```python
from build123d import *

# Parameters (mm, degrees)
BOSS_EXTRUDE1_DEPTH             = 5
F_3_0_3_DIAMETER_HOLE1_D        = 3
F_3_0_3_DIAMETER_HOLE1_DEPTH    = 6
F_3_0_3_DIAMETER_HOLE1_TIP      = 0.901290929
SKETCH6_W                       = 36
SKETCH6_H                       = 124
CUT_EXTRUDE1_DEPTH              = 3
SKETCH9_W                       = 20
SKETCH9_H                       = 45
CUT_EXTRUDE3_DEPTH              = 6
M3X0_5_TAPPED_HOLE1_D           = 2.5
M3X0_5_TAPPED_HOLE1_DEPTH       = 5
M3X0_5_TAPPED_HOLE1_CSINK_D     = 3.05
M3X0_5_TAPPED_HOLE1_CSINK_ANGLE = 90


with BuildPart() as part:
    # Sketch3 → Boss-Extrude1 (new body)
    with BuildSketch(Plane(origin=(0, -40, 0), x_dir=(-1, 0, 0), z_dir=(0, -1, 0))):
        Polygon((18.468579028, -110), (85.532661839, -110), (127, -68.532661839), (127, -18.529510204), (108.472719443, 10), (-4.471478576, 10), (-23, -18.531420972), (-23, -68.531420972), align=None)
    extrude(amount=BOSS_EXTRUDE1_DEPTH)

    # Ø3.0 (3) Diameter Hole1
    with Locations(Plane(origin=(0, -45, 0), x_dir=(-1, 0, 0), z_dir=(0, -1, 0))):
        with Locations((8.156954779, -77.608240604), (95.838195646, -77.608240604), (103.995150425, 0), (0, 0)):
            Hole(F_3_0_3_DIAMETER_HOLE1_D / 2, depth=F_3_0_3_DIAMETER_HOLE1_DEPTH)
            with Locations((0, 0, -(F_3_0_3_DIAMETER_HOLE1_DEPTH + F_3_0_3_DIAMETER_HOLE1_TIP / 2))):  # 118° drill point
                Cone(0, F_3_0_3_DIAMETER_HOLE1_D / 2, F_3_0_3_DIAMETER_HOLE1_TIP, mode=Mode.SUBTRACT)

    # Sketch6 → Cut-Extrude1 (cut)
    with BuildSketch(Plane(origin=(0, -45, 0), x_dir=(-1, 0, 0), z_dir=(0, -1, 0))):
        with Locations((52, -55)):
            Rectangle(SKETCH6_W, SKETCH6_H)
    extrude(amount=-CUT_EXTRUDE1_DEPTH, mode=Mode.SUBTRACT)

    # Sketch9 → Cut-Extrude3 (cut, through all)
    with BuildSketch(Plane(origin=(0, -45, 0), x_dir=(-1, 0, 0), z_dir=(0, -1, 0))):
        with Locations((4, -45.108240604)):
            Rectangle(SKETCH9_W, SKETCH9_H)
    cut_extrude3 = extrude(amount=-CUT_EXTRUDE3_DEPTH, mode=Mode.SUBTRACT)

    # Mirror1: Cut-Extrude3 across plane
    add(cut_extrude3.mirror(Plane.ZY.offset(52)), mode=Mode.SUBTRACT)

    # M3x0.5 Tapped Hole1
    with Locations(Plane(origin=(0, -40, 0), x_dir=(1, 0, 0), z_dir=(0, 1, 0))):
        with Locations((-8.156954779, 0), (-95.838195646, 0)):
            CounterSinkHole(M3X0_5_TAPPED_HOLE1_D / 2, M3X0_5_TAPPED_HOLE1_CSINK_D / 2, depth=M3X0_5_TAPPED_HOLE1_DEPTH, counter_sink_angle=M3X0_5_TAPPED_HOLE1_CSINK_ANGLE)


solid = part.part
```
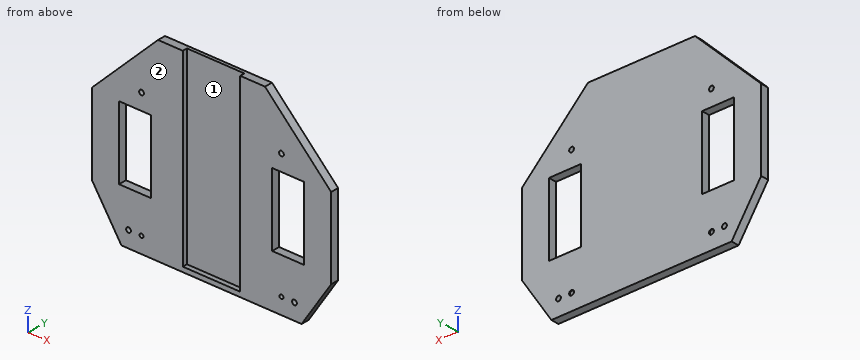
CAD build for the part. Positions are in the model's coordinates, mm. Face numbers are marked on the shaded views. A direction names the side the tool comes from. Round coordinates to 2 decimals unless told otherwise and drop trailing zeros. Order: outer loops, then holes, each group sorted by start corner. A loop starts at its lowest first (then second) coordinate and runs counter-clockwise, first axis right, second up.
Q1. Slice it at C-C (y = -44.25). State how many separate pieces and enclosed holes the cut face has, and give its area (3 significant figures).
Q2. Slice it at D-D (z = 102). Write the cut outline in (x, y), and give its area (3 significant figures).
Q3. Drop flat-ended pins along their axis: pin 1 (1 mm diameter, centred on y = -41, z = 86, fed in from +X); pin 2 (2.5 mm diameter, centred on x = -104.5, y = -41.5, fed in from +Z); pin 3 (5 mm diameter, centred on x = -8.16, z = 77.61, fed in from +Y); pin 4 (2 mm diameter, centred on x = 4, y = -42.5, fed in from +Z). Give the stop position or say it passes through.
Q4. Slice it at A-A (z = 36). Write the cut outline in (x, y), and give its area (3 significant figures).
Q5. Slice it at B-B (x = -56). Write the cut outline in (y, z).
Q6. Wall check: L1, parallel to X at y = -40.8, z = 35; L2, parallel to X at y = -43.1, z = 34.5; L3, parallel to X at y = -44.05, z = 68. Give the ranges that are in metal, low to high.
Q7. Which spindle directions (+Z, -Z, +X, -X, +Y, -Y) get a long thin tool onto all of the face, cutting with end or side? Do the marked faces 1 and 2. Say none if no direction does.
Results below:
1. separate pieces: 1
1. enclosed holes: 8
1. area: 9,700 mm2
2. outline: (-93.53, -45) - (-70, -45) - (-70, -42) - (-34, -42) - (-34, -45) - (-10.47, -45) - (-10.47, -40) - (-93.53, -40) - close
2. area: 307 mm2
3. pin 1: stops at x = 6.03
3. pin 2: stops at z = 92.28
3. pin 3: stops at y = -40
3. pin 4: stops at z = 88.53
4. outline: (-127, -45) - (-110, -45) - (-110, -40) - (-127, -40) - close; (-90, -45) - (-70, -45) - (-70, -42) - (-34, -42) - (-34, -45) - (-14, -45) - (-14, -40) - (-90, -40) - close; (6, -45) - (23, -45) - (23, -40) - (6, -40) - close
4. area: 442 mm2
5. outline: (-45, -10) - (-40, -10) - (-40, 110) - (-42, 110) - (-42, -7) - (-45, -7) - close
6. L1: x = -127 to -110, -90 to -14, 6 to 23
6. L2: x = -127 to -110, -90 to -70, -34 to -14, 6 to 23
6. L3: x = -127 to -70, -34 to 23
7. face 1: +Z, -Y
7. face 2: +Z, -Z, +X, -X, -Y
